Autodesk Inventor part; units mm, degrees
ref_plane "YZ Plane" through (0, 0, 0) normal (1, 0, 0) x (0, 1, 0)
ref_plane "XZ Plane" through (0, 0, 0) normal (0, 1, 0) x (-1, 0, 0)
ref_plane "XY Plane" through (0, 0, 0) normal (0, 0, 1) x (1, 0, 0)
sketch "Sketch1" plane through (0, 0, 0) normal (0, 1, 0) x (-1, 0, 0)
  line L0 (0, 0) -> (55.5, 0)
  line L1 (55.5, 0) -> (55.5, 55.5)
  line L2 (55.5, 55.5) -> (0, 55.5)
  line L3 (0, 55.5) -> (0, 0)
  line L4 (-1, 60.5) -> (56.5, 60.5)
  line L5 (60.5, 56.5) -> (60.5, -1)
  line L6 (56.5, -5) -> (-1, -5)
  line L7 (-5, -1) -> (-5, 56.5)
  arc A0 (60.5, 56.5) -> (56.5, 60.5) centre (56.5, 56.5) ccw
  arc A1 (56.5, -5) -> (60.5, -1) centre (56.5, -1) ccw
  arc A2 (-5, -1) -> (-1, -5) centre (-1, -1) ccw
  arc A3 (-1, 60.5) -> (-5, 56.5) centre (-1, 56.5) ccw
  dimension "d0" = 55.5
  dimension "d1" = 55.5
  dimension "d2" = 5
  dimension "d3" = 4
extrude "Extrusion1" add sketch "Sketch1" along normal blind 4
sketch "Sketch2" plane through (0, 0, 0) normal (0, -1, 0) x (1, 0, 0)
  line L0 (1, -5) -> (-56.5, -5)
  arc A0 (1, -5) -> (5, -1) centre (1, -1) ccw
  line L1 (5, 56.5) -> (5, -1)
  arc A1 (5, 56.5) -> (1, 60.5) centre (1, 56.5) ccw
  line L2 (-56.5, 60.5) -> (1, 60.5)
  arc A2 (-56.5, 60.5) -> (-60.5, 56.5) centre (-56.5, 56.5) ccw
  line L3 (-60.5, -1) -> (-60.5, 56.5)
  arc A3 (-60.5, -1) -> (-56.5, -5) centre (-56.5, -1) ccw
  line L4 (0, 0) -> (0, 55.5)
  line L5 (-55.5, 0) -> (0, 0)
  line L6 (-55.5, 55.5) -> (-55.5, 0)
  line L7 (0, 55.5) -> (-55.5, 55.5)
  line L8 (-77.75, 77.75) -> (22.25, 77.75) construction
  line L9 (22.25, 77.75) -> (22.25, -22.25) construction
  line L10 (22.25, -22.25) -> (-77.75, -22.25) construction
  line L11 (-77.75, -22.25) -> (-77.75, 77.75) construction
  line L12 (-77.75, 77.75) -> (22.25, -22.25) construction
  line L13 (22.25, 77.75) -> (-77.75, -22.25) construction
  circle A4 centre (10.7227, 66.2227) radius 2.75
  arc A5 (17.617, 59.3284) -> (3.8284, 73.117) centre (10.7227, 66.2227) ccw
  arc A6 (5, 56.5) -> (1, 60.5) centre (1, 56.5) ccw
  line L14 (17.617, 59.3284) -> (5, 46.7114)
  line L15 (3.8284, 73.117) -> (-8.7886, 60.5)
  line L16 (-59.3284, 73.117) -> (-46.7114, 60.5)
  arc A7 (-59.3284, 73.117) -> (-73.117, 59.3284) centre (-66.2227, 66.2227) ccw
  circle A8 centre (-66.2227, 66.2227) radius 2.75
  line L17 (-73.117, 59.3284) -> (-60.5, 46.7114)
  line L18 (-73.117, -3.8284) -> (-60.5, 8.7886)
  arc A9 (-73.117, -3.8284) -> (-59.3284, -17.617) centre (-66.2227, -10.7227) ccw
  circle A10 centre (-66.2227, -10.7227) radius 2.75
  line L19 (-59.3284, -17.617) -> (-46.7114, -5)
  line L20 (3.8284, -17.617) -> (-8.7886, -5)
  arc A11 (3.8284, -17.617) -> (17.617, -3.8284) centre (10.7227, -10.7227) ccw
  circle A12 centre (10.7227, -10.7227) radius 2.75
  line L21 (17.617, -3.8284) -> (5, 8.7886)
  point P0 (-27.75, 27.75)
  dimension "d6" = 100
  dimension "d7" = 100
  dimension "d8" = 5.5
  dimension "d9" = 7
  dimension "d12" = 360
extrude "Extrusion2" add sketch "Sketch2" along normal blind 4 contours A0 L1 L21 A11 L20 L0 | L0 A3 L3 A2 L2 A1 L1 A0 | L19 A9 L18 L3 A3 L0 | L1 A1 L2 L15 A5 L14 | L17 A7 L16 L2 A2 L3 | L5 L6 L7 L4
sketch "Sketch3" plane through (0, 0, 0) normal (0, 1, 0) x (1, 0, 0)
  line L0 (-52.25, -52.25) -> (-3.25, -52.25) construction
  line L1 (-3.25, -52.25) -> (-3.25, -3.25) construction
  line L2 (-3.25, -3.25) -> (-52.25, -3.25) construction
  line L3 (-52.25, -3.25) -> (-52.25, -52.25) construction
  line L4 (-52.25, -52.25) -> (-52.25, -55.5) construction
  line L5 (-52.25, -52.25) -> (-55.5, -52.25) construction
  line L6 (-55.5, -55.5) -> (-55.5, 0) construction
  line L7 (-3.25, -3.25) -> (0, -3.25) construction
  line L8 (0, 0) -> (0, -55.5) construction
  line L9 (-3.25, -3.25) -> (-3.25, 0) construction
  line L10 (-55.5, 0) -> (0, 0) construction
  line L11 (0, -55.5) -> (-55.5, -55.5)
  circle A0 centre (-52.25, -52.25) radius 3.25
  circle A1 centre (-52.25, -3.25) radius 3.25
  circle A2 centre (-3.25, -3.25) radius 3.25
  circle A3 centre (-3.25, -52.25) radius 3.25
  line L12 (-55.5, 0) -> (0, 0)
  line L13 (-55.5, -55.5) -> (-55.5, 0)
  line L14 (0, -55.5) -> (-55.5, -55.5)
  line L15 (0, 0) -> (0, -55.5)
  point P0 (-3.25, 0)
  point P1 (0, -3.25)
  point P2 (0, -52.25)
  point P3 (-3.25, -55.5)
  point P4 (-55.5, -3.25)
  point P5 (-52.25, 0)
  dimension "d16" = 49
  dimension "d17" = 49
extrude "Extrusion3" add sketch "Sketch3" along normal blind 2.3 contours L11 A3 L15 | A3 | L11 L13 A0 | A0 | A2 | A2 L12 L15 | L13 L12 A1 | A1
sketch "Sketch4" plane through (0, 2.3, 0) normal (0, 1, 0) x (1, 0, 0)
  arc A0 (0, -52.25) -> (-3.25, -55.5) centre (-3.25, -52.25) ccw
  line L0 (0, -3.25) -> (0, -52.25)
  arc A1 (-3.25, 0) -> (0, -3.25) centre (-3.25, -3.25) ccw
  line L1 (-52.25, 0) -> (-3.25, 0)
  arc A2 (-55.5, -3.25) -> (-52.25, 0) centre (-52.25, -3.25) ccw
  line L2 (-55.5, -52.25) -> (-55.5, -3.25)
  arc A3 (-52.25, -55.5) -> (-55.5, -52.25) centre (-52.25, -52.25) ccw
  line L3 (-3.25, -55.5) -> (-52.25, -55.5)
  point P0 (0, 0)
extrude "Extrusion4" cut sketch "Sketch4" against normal blind 3
sketch "Sketch5" plane through (0, 2.3, 0) normal (0, 1, 0) x (1, 0, 0)
  line L0 (0, 0) -> (0, -3.25)
  line L1 (-3.25, 0) -> (0, 0)
  arc A0 (-3.25, 0) -> (0, -3.25) centre (-3.25, -3.25) ccw
  arc A1 (0, -52.25) -> (-3.25, -55.5) centre (-3.25, -52.25) ccw
  line L2 (0, -55.5) -> (-3.25, -55.5)
  line L3 (0, -52.25) -> (0, -55.5)
  line L4 (-52.25, -55.5) -> (-55.5, -55.5)
  arc A2 (-52.25, -55.5) -> (-55.5, -52.25) centre (-52.25, -52.25) ccw
  line L5 (-55.5, -55.5) -> (-55.5, -52.25)
  arc A3 (-55.5, -3.25) -> (-52.25, 0) centre (-52.25, -3.25) ccw
  line L6 (-55.5, 0) -> (-52.25, 0)
  line L7 (-55.5, -3.25) -> (-55.5, 0)
  circle A4 centre (-52.25, -52.25) radius 1
  arc A5 (-55.5, -3.25) -> (-52.25, 0) centre (-52.25, -3.25) ccw
  circle A6 centre (-52.25, -3.25) radius 1
  arc A7 (-3.25, 0) -> (0, -3.25) centre (-3.25, -3.25) ccw
  circle A8 centre (-3.25, -3.25) radius 1
  circle A9 centre (-3.25, -52.25) radius 1
  dimension "d23" = 2
  dimension "d24" = 2
  dimension "d25" = 2
  dimension "d26" = 2
extrude "Extrusion5" cut sketch "Sketch5" against normal up to next contours A4 | A6 | A8 | A9
chamfer "Chamfer1" distance 1 angle 45 4 edges at (-53.25, 2.3, 52.25) (-53.25, 2.3, 3.25) (-4.25, 2.3, 52.25) (-4.25, 2.3, 3.25)
equation "\"d24\" = d23"
equation "\"d25\" = d23"
equation "\"d26\" = d23"
properties part number "Drok L298 DC Motor Driver Mount"
For this review, take the finished solid that the model builds, in its own axes (mm). A direction names the side the tool comes from. Give positions to 0.01 mm unless a question says otherwise; leave off trailing zeros. Loops run counter-clockwise (first coordinate to the right, second up) from the corner with the lowest first, then second, coordinate; pieces in that order, holes last. Notation, with made-up numbers: M -11.75,-17.5 L -1.75,-17.5 A19 cw -1.75,-2.5 Z; hole C -30.75,-21 d6. An arc over 180 degrees is marked long. Put each result on its own line as item: value. Start each with the question number.
(1) The part is to be moulded in two halves that separate along X. For faces 4 (the flat face through (-28, -4, 28)), 5 (the flat face through (11.4, -1.97, 53.11)), 6 (the flat face through (0, 2, 28)), say which applies: +X half, -X half, draft (parallel to the pull), parting line (faces both ways), or undercut.
(2) Wall thickness on L1, parallel to X at y = -0.5, z = -9; L2, parallel to Z at x = -23, y = 0.5; L3, parallel to Z at x = 13, y = -0.25: over which ranges is each line inside the solid? List them lowest first.
(3) Add section A-A, the plane z = -12. Write out the cut boundary in (x, y).
(4) Machinability: for faces 1 (the flat face through (-62, 0, 65)), 2 (the flat face through (5, 0, 27)), 3 (the flat face through (-53.11, -1.97, 66.9)), which of the approach directions +Z, -Z, +X, -X, +Y, -Y give a long, thin tool a straight path to every point of the face, cutting with its end or side? Answer none if there is none.
(5) Add section C-C, the plane z = 37. Write out the cut boundary in (x, y).
(6) Add section B-B, the plane x = -25.5. Write out the cut boundary in (y, z).
(7) For pin 1 (7 mm diameter, centred on x = -4.5, z = 4.5, fed in from +Y); pin 2 (4 mm diameter, centred on y = 1.5, z = 17.5, fed in from +X); pin 3 (4 mm diameter, centred on y = -2, z = 39, fed in from -X), all flat-tipped, find the tip position at first contact; note any pin that passes through.
Result:
1. face 4: draft
1. face 5: +X half
1. face 6: undercut
2. L1: x = -75.82 to -68.37, -64.08 to -50.71, -4.79 to 8.58, 12.87 to 20.32
2. L2: z = -5 to 0, 55.5 to 60.5
2. L3: z = -20.2 to -12.26, -9.18 to 0.79, 54.71 to 64.68, 67.76 to 75.7
3. outline: M -75.89,-4 L -68.66,-4 L -68.66,0 L -75.89,0 Z; M -63.79,-4 L -53.71,-4 L -53.71,0 L -63.79,0 Z; M -1.79,-4 L 8.29,-4 L 8.29,0 L -1.79,0 Z; M 13.16,-4 L 20.39,-4 L 20.39,0 L 13.16,0 Z
4. face 1: +Z, -X, +Y
4. face 2: +X, +Y
4. face 3: +Z, +Y, -Y
5. outline: M -60.5,-4 L 5,-4 L 5,4 L 0,4 L 0,-0.7 L -55.5,-0.7 L -55.5,4 L -60.5,4 Z
6. outline: M -4,-5 L 4,-5 L 4,0 L -0.7,0 L -0.7,55.5 L 4,55.5 L 4,60.5 L -4,60.5 Z
7. pin 1: stops at y = 2.3
7. pin 2: stops at x = 5
7. pin 3: stops at x = -60.5
